Geometry check sheet. Reference: drawing and pictorial views, mm from the part's lowest x, y, z. A direction names the side the tool comes from. Give positions to 0.01 mm unless a question says otherwise; leave off trailing zeros. Loops run counter-clockwise (first coordinate to the right, second up) from the corner with the lowest first, then second, coordinate; pieces in that order, holes last. Notation, with made-up numbers: (88, -19) - (146, -19) arc R32 ccw to (146, 8) - close; hole circle Ø6 at (-8.75, 68.25). An arc over 180 degrees is marked (long way). Answer in a Markdown table with one row per item. Add a question column.
(1) Set-up check for the marked faces 4, 5 and 6: record each of +Z, -Z, +X, -X, +Y, -Y from which the full face is reachable in a straight line by a thin tool's end or side.
(2) Draft check along X on the marked faces 1, 2 and 3. Enter one of: released by +X, released by -X, zero draft, split by the parting line, or undercut.
(3) Thickness scan on L1, parallel to Y at x = 15, z = 3.25; L2, parallel to Y at x = 18.5, z = 14.5. Record the ranges inside material, lowest first.
(4) Sectioned sample at D-D on z = 14. Enter the section's corners in (x, y), then the cut area to 3 significant figures.
(5) Go/stop test with flat-tipped pins: P1, Ø7, axis at y = 18.5, z = 16, coming from the +X side; P2, Ø5, axis at x = 45, y = 15, coming from the +Z side; P3, Ø4, axis at x = 51, z = 13.5, coming from the +Y side; P4, Ø12, axis at x = 23, z = 14, coming from the +Y side. Record where each tip stops, or that it passes through.
(6) Sectioned sample at A-A on y = 45. Enter the section's corners in (x, z).
(7) Sectioned sample at C-C on z = 2. Enter the section's corners in (x, y), then the cut area to 3 significant figures.
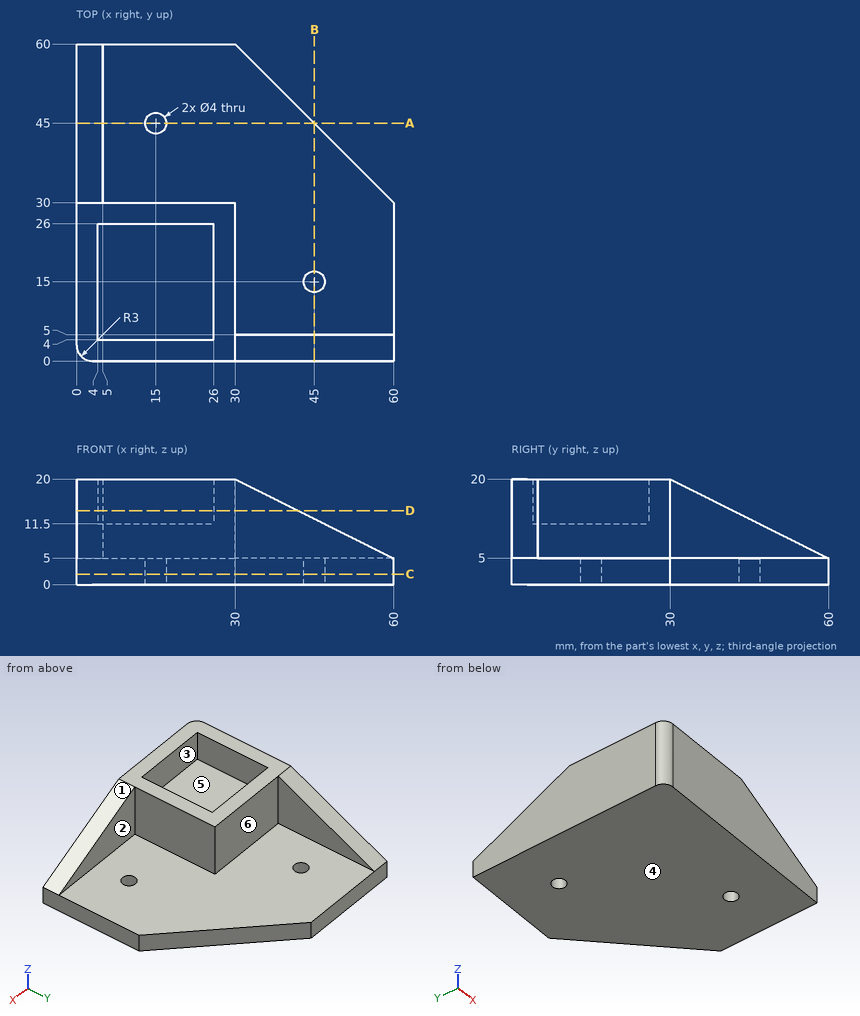
Reply:
| question | item | result |
|---|---|---|
| 1 | face 4 | -Z, +X, -X, +Y, -Y |
| 1 | face 5 | +Z |
| 1 | face 6 | +Z, +X, +Y |
| 2 | face 1 | released by +X |
| 2 | face 2 | zero draft |
| 2 | face 3 | undercut |
| 3 | L1 | 0 to 43, 47 to 60 |
| 3 | L2 | 0 to 4, 26 to 30 |
| 4 | outline | (0, 3) arc R3 ccw to (3, 0) - (42, 0) - (42, 5) - (30, 5) - (30, 30) - (5, 30) - (5, 42) - (0, 42) - close; hole (4, 4) - (26, 4) - (26, 26) - (4, 26) - close |
| 4 | area | 534 mm^2 |
| 5 | P1 | x = 30 |
| 5 | P2 | z = 5 |
| 5 | P3 | through |
| 5 | P4 | y = 30 |
| 6 | outline | (0, 0) - (13, 0) - (13, 5) - (5, 5) - (5, 12.5) - (0, 12.5) - close; (17, 0) - (45, 0) - (45, 5) - (17, 5) - close |
| 7 | outline | (0, 3) arc R3 ccw to (3, 0) - (60, 0) - (60, 30) - (30, 60) - (0, 60) - close; hole circle Ø4 at (15, 45); hole circle Ø4 at (45, 15) |
| 7 | area | 3,120 mm^2 |
